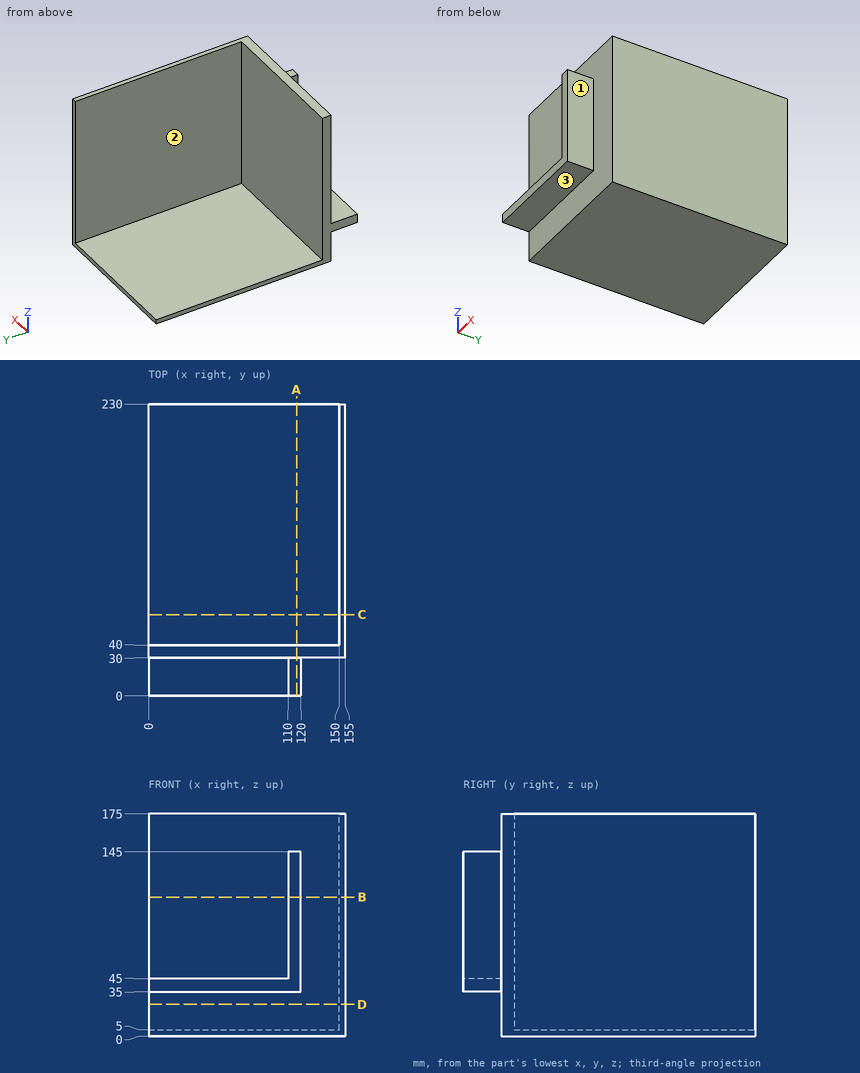
Could you check a few things on this drawing? It's one solid part, dimensions in mm from its lowest x, y, z. A direction names the side the tool comes from. Round coordinates to 2 decimals unless told otherwise and drop trailing zeros. Order: outer loops, then holes, each group sorted by start corner. A loop starts at its lowest first (then second) coordinate and runs counter-clockwise, first axis right, second up. Notation, with made-up numbers: M 38.5,66 L 73.5,66 A18 ccw 73.5,86 Z; hole C 78.25,-32 d7. An arc over 180 degrees is marked long. One line per question, with ' | ' between items.
1) I'm going to push flat-ended pins straight in: pin 1 Ø24 at (x, y) = (90, 17.5) entering from -Z; pin 2 Ø5 at (x, y) = (132.5, 154) entering from +Z; pin 3 Ø10 at (x, z) = (89, 59) entering from -Y. Where does each tip first touch, or does it pass through?
Checked values:
pin 1: stops at z = 35 | pin 2: stops at z = 5 | pin 3: stops at y = 30
2) Imagine slicing it at D-D, the plane z = 25. Write out the boundary of the cut face in (x, y), plus the area to 3 significant figures.
Checked values:
outline: M 0,30 L 155,30 L 155,230 L 150,230 L 150,40 L 0,40 Z | area: 2,500 mm²
3) Imagine slicing it at A-A, the plane x = 116.5. Write out the boundary of the cut face in (y, z), plus the area to 3 significant figures.
Checked values:
outline: M 0,35 L 30,35 L 30,0 L 230,0 L 230,5 L 40,5 L 40,175 L 30,175 L 30,145 L 0,145 Z | area: 6,000 mm²
4) Imagine slicing it at B-B, the plane z = 109.5. Write out the boundary of the cut face in (x, y), plus the area to 3 significant figures.
Checked values:
outline: M 0,30 L 110,30 L 110,0 L 120,0 L 120,30 L 155,30 L 155,230 L 150,230 L 150,40 L 0,40 Z | area: 2,800 mm²
5) I need wall thicknesses on line 1 (X direction, y = 153, z = 8.5); line 2 (Y direction, x = 20.5, z = 43.5); line 3 (Y direction, x = 73.5, z = 54.5). Which ranges of each line are inside material? Lowest first, please.
Checked values:
line 1: x = 150 to 155 | line 2: y = 0 to 40 | line 3: y = 30 to 40
6) On a 3-axis mill with a long thin cutter (end or side, diameter ignored), from which of +Z, -Z, +X, -X, +Y, -Y can I reach the whole of each face in a straight line? I mean the marked faces 1, 2 and 3. Say none if no direction works.
Checked values:
face 1: +Z, -Z, +X, -Y | face 2: +Z, -X, +Y | face 3: -Z, +X, -X, -Y
7) Imagine slicing it at C-C, the plane y = 64. Write out the boundary of the cut face in (x, z), plus the area to 4 significant figures.
Checked values:
outline: M 0,0 L 155,0 L 155,175 L 150,175 L 150,5 L 0,5 Z | area: 1,625 mm²
